Part model, mm, in its own coordinate system. Face numbers are marked on the shaded views. A direction names the side the tool comes from. Give positions to 0.01 mm unless a question says otherwise; leave off trailing zeros. Write each loop counter-clockwise with the first axis right and the second up, starting at its lowest first coordinate (ties: lowest second). Pieces come first, ordered by that corner, then holes. Notation, with made-up numbers: M 34.5,69 L 85.5,69 A28 cw 85.5,94 Z; hole C 6,-34 d2. An arc over 180 degrees is marked long. Answer as CSV lines item,"result". Start each with the question number.
Item 1: Pin check, flat tips, straight feed: pin 1 (8 mm diameter, centred on y = 63.5, z = 51.5, fed in from -X); pin 2 (3.5 mm diameter, centred on y = 5.5, z = 49, fed in from +X); pin 3 (12 mm diameter, centred on y = 22, z = 52, fed in from +X). Stop position of each tip, or through.
Item 2: Band-saw the part on C-C, the plane y = 43. List the corners of the cut face in (x, z), then the cut area to 3 significant figures.
Item 3: Band-saw the part on D-D, the plane x = 270.5. List the corners of the cut face in (y, z), then the cut area to 3 significant figures.
Item 4: Band-saw the part on A-A, the plane x = 197. List the corners of the cut face in (y, z).
Item 5: 3-axis set-ups, long thin cutter, end or side, ignore diameter. For the marked faces 1 and 2: which of +Z, -Z, +X, -X, +Y, -Y reach the whole face in a straight line?
Item 6: Band-saw the part on B-B, the plane z = 25. List the corners of the cut face in (x, y), then the cut area to 3 significant figures.
Item 7: Two-plate mould, pull along X, no slides. Class the marked faces 3, 4 and 5: +X half, -X half, draft (parallel to the pull), parting line (faces both ways), or undercut.
Item 8: Wall check: L1, parallel to Z at x = 102.5, y = 59; L2, parallel to Z at x = 163.5, y = 5; L3, parallel to Y at x = 16.5, z = 78.5. Give the ranges that are in metal, low to high. Write a range as from..to.
Autodesk Fusion 360 part; units mm, degrees
sketch "hopper" plane through (0, 0, 0) normal (0, 0, 1) x (1, 0, 0)
  line L0 (0, 0) -> (254, 0)
  line L1 (0, 0) -> (-8.4458, 0)
  line L2 (-8.4458, 0) -> (-50, 75)
  line L3 (-50, 75) -> (325, 75)
  line L4 (325, 75) -> (254, 0)
  dimension "d4" = 375
  dimension "d5" = 61.011
  dimension "d6" = 46.569
  dimension "d7" = 75
  dimension "d19" = 262.4458
extrude "Extrude1" add sketch "hopper" along normal blind 100
shell "Shell1" thickness 10 removed faces 1 at (75, 75, 33.3333)
sketch "tube slot" plane through (0, 0, 0) normal (0, 1, 0) x (1, 0, 0)
  line L0 (10, -50) -> (241.775, -50)
  line L1 (241.775, -50) -> (241.775, -46.75)
  line L2 (241.775, -46.75) -> (10, -46.75)
  line L3 (10, -46.75) -> (10, -50)
  line L4 (-8.4458, -100) -> (254, -100)
  line L5 (254, 0) -> (254, -100)
  dimension "d11" = 231.775
  dimension "d12" = 3.25
  dimension "d15" = 50
  dimension "d16" = 12.225
extrude "Extrude2" cut sketch "tube slot" along normal blind 30
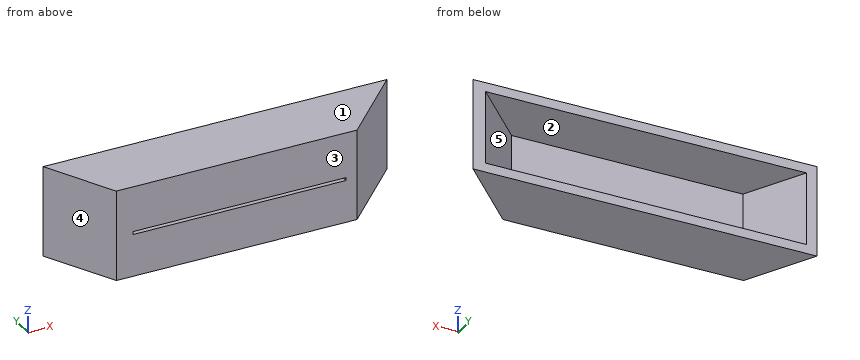
Output:
1,pin 1,"x = -45.84"
1,pin 2,"x = 260.86"
1,pin 3,"x = 280.51"
2,outline,"M -32.27,0 L 294.71,0 L 294.71,100 L -32.27,100 Z; hole M -20.84,10 L 280.94,10 L 280.94,90 L -20.84,90 Z"
2,area,"8,560 mm²"
3,outline,"M 17.43,0 L 75,0 L 75,10 L 31.98,10 L 31.98,90 L 75,90 L 75,100 L 17.43,100 Z"
3,area,"2,320 mm²"
4,outline,"M 0,0 L 75,0 L 75,10 L 10,10 L 10,46.75 L 0,46.75 Z; M 0,50 L 10,50 L 10,90 L 75,90 L 75,100 L 0,100 Z"
5,face 1,"+Z, +X, -X, +Y, -Y"
5,face 2,"+Y"
6,outline,"M -50,75 L -8.45,0 L 254,0 L 325,75 L 311.23,75 L 249.7,10 L -2.55,10 L -38.57,75 Z"
6,area,"4,340 mm²"
7,face 3,"draft"
7,face 4,"-X half"
7,face 5,"undercut"
8,L1,"0..10, 90..100"
8,L2,"0..46.75, 50..100"
8,L3,"0..10"
